from build123d import *

# Parameters (mm, degrees)
BOSS_EXTRUDE1_DEPTH = 18
FILLET1_R           = 5


with BuildPart() as part:
    # Sketch1 → Boss-Extrude1 (new body)
    with BuildSketch(Plane(origin=(0, 0, 0), x_dir=(1, 0, 0), z_dir=(0, 1, 0))):
        with BuildLine():
            Line((-455.426852277, -314.819999892), (-38.000000187, -314.819999892))
            ThreePointArc((-38.000000187, -314.819999892), (-35.878679843, -313.941320236), (-35.000000187, -311.819999892))
            Line((-35.000000187, -311.819999892), (-35.000000187, -290.999999892))
            Line((-35.000000187, -290.999999892), (34.999999813, -290.999999892))
            Line((34.999999813, -290.999999892), (34.999999813, -311.819999892))
            ThreePointArc((34.999999813, -311.819999892), (35.87867947, -313.941320236), (37.999999813, -314.819999892))
            Line((37.999999813, -314.819999892), (455.426851904, -314.819999892))
            ThreePointArc((455.426851904, -314.819999892), (479.472561657, -276.823612404), (500.355543579, -237.001223154))
            Line((500.355543579, -237.001223154), (291.642117601, 124.501034862))
            ThreePointArc((291.642117601, 124.501034862), (289.820498525, 125.898812341), (287.54404139, 125.599111073))
            Line((287.54404139, 125.599111073), (269.513392244, 115.189110935))
            Line((269.513392244, 115.189110935), (234.513392244, 175.8108892))
            Line((234.513392244, 175.8108892), (252.544041237, 186.220889249))
            ThreePointArc((252.544041237, 186.220889249), (253.941818715, 188.042508325), (253.642117448, 190.318965461))
            Line((253.642117448, 190.318965461), (44.928691409, 551.821223582))
            ThreePointArc((44.928691409, 551.821223582), (-7e-08, 553.647225338), (-44.928691549, 551.821223601))
            Line((-44.928691549, 551.821223601), (-253.642117655, 190.318965363))
            ThreePointArc((-253.642117655, 190.318965363), (-253.941818922, 188.042508228), (-252.544041443, 186.220889153))
            Line((-252.544041443, 186.220889153), (-234.513392501, 175.810889132))
            Line((-234.513392501, 175.810889132), (-269.513392501, 115.189110868))
            Line((-269.513392501, 115.189110868), (-287.544041036, 125.599110653))
            ThreePointArc((-287.544041036, 125.599110653), (-289.820498172, 125.89881192), (-291.642117248, 124.50103444))
            Line((-291.642117248, 124.50103444), (-500.355543515, -237.001224077))
            ThreePointArc((-500.355543515, -237.001224077), (-479.472561775, -276.823612847), (-455.426852277, -314.819999892))
        make_face()
    extrude(amount=BOSS_EXTRUDE1_DEPTH)

    # Fillet1
    fillet1_edges = [part.edges().sort_by_distance(p)[0] for p in [
        (-269.513392501, 9, -115.189110868),
        (-234.513392501, 9, -175.810889132),
        (234.513392244, 9, -175.8108892),
        (269.513392244, 9, -115.189110935),
        (34.999999813, 9, 290.999999892),
        (-35.000000187, 9, 290.999999892),
    ]]
    fillet(fillet1_edges, radius=FILLET1_R)


solid = part.part
Geometry check sheet. Reference: the model listing, model coordinates, mm. Give positions to 0.01 mm unless a question says otherwise; leave off trailing zeros. Loops run counter-clockwise (first coordinate to the right, second up) from the corner with the lowest first, then second, coordinate; pieces in that order, holes last.
(1) Section check B-B on x = 90. Record the cut outline in (y, z).
From the geometry:
outline: (0, -473.76) - (18, -473.76) - (18, 314.82) - (0, 314.82) - close
(2) Depth check by flat-ended pin: pin 1 Ø9 at (x, y) = (12, 9.5) entering from +Z; pin 2 Ø3 at (x, y) = (-101, 8) entering from -Z; pin 3 Ø5 at (y, z) = (13, -422.5) entering from +X. Enter the tip coordinate at first touch or a pass-through.
From the geometry:
pin 1: stops at z = 291
pin 2: stops at z = -457.3
pin 3: stops at x = 121.04
(3) Thickness scan on L1, parallel to X at y = 9.75, z = -175; L2, parallel to Z at x = 219, y = 10.75; L3, parallel to X at y = 7.25, z = 161.5. Record the ranges inside material, lowest first.
From the geometry:
L1: x = -236.45 to 236.45
L2: z = -250.32 to 314.82
L3: x = -456.76 to 456.76
(4) Section check C-C on z = -35. Record the cut outline in (x, y), then the cut area to 3 significant figures.
From the geometry:
outline: (-343.32, 0) - (343.32, 0) - (343.32, 18) - (-343.32, 18) - close
area: 12,400 mm2
